Can you work these out from the model? Positions are in its coordinate system, mm. A direction names the side the tool comes from. Give positions to 0.01 mm unless a question says otherwise; leave off trailing zeros. Loops run counter-clockwise (first coordinate to the right, second up) from the corner with the lowest first, then second, coordinate; pieces in that order, holes last. Notation, with made-up numbers: (62, 7.25) -> (91, 7.25) arc R17 ccw to (91, 16.25) -> close; hole circle Ø9 at (71.25, 30). An arc over 180 degrees is marked (long way). Return JSON: item names as keys, results as strings. Group by question number.
Q1. Which directions (+Z, -Z, +X, -X, +Y, -Y) give clear straight access to the entire face, cutting with the end or side of a thin tool? Please do faces 5 (the cylindrical face through (-36.495, 3.486, -27.382)), 6 (the flat face through (0, 3, 36.5)), 7 (the flat face through (-18.958, 2.282, 1.44)), 8 (the cylindrical face through (17.29, 3.49, 33.04)).
Q2. I need wall thicknesses on line 1 along Z through (x, y) = (6, 4.3); line 2 along Z through (x, y) = (-15.5, 2.25); line 3 along Y through (x, z) = (-44, -10.5). Which ranges of each line are inside material? Lowest first, please. Write a range as [from, to].
Q3. Thinking about a two-plate mould opening in X: for faces 1 (the flat face through (0, 3, -36.5)), 2 (the cylindrical face through (33.535, 2.218, -19.087)), 3 (the cylindrical face through (18.945, 2.218, 19.066)), 4 (the flat face through (40.18, 0.74, -0.58)), which applies, pulls with the +X half, pulls with the -X half, needs draft (parallel to the pull), parting line crosses it, or undercut?
Q4. Suppose I cut it at C-C, the plane z = -17.5. Please give me the cut outline in (x, y), and give its area (3 significant figures).
Q5. Suppose I cut it at B-B, the plane y = 3.8. Please give me the cut outline in (x, z).
Q6. Suppose I cut it at A-A, the plane x = 4.5. Please give me the cut outline in (y, z), and give its area (3 significant figures).
Q7. Suppose I cut it at D-D, the plane z = 6.5. Please give me the cut outline in (x, y), and give its area (3 significant figures).
Q8. Will these pins go through, and if not, where does the flat tip stop? pin 1 (1 mm diameter, centred on x = 29.5, y = 4, fed in from +Z); pin 2 (2.5 mm diameter, centred on x = -6, y = 3, fed in from -Z); pin 3 (2 mm diameter, centred on y = 3, z = 3, fed in from -X).
Autodesk Inventor part; units mm, degrees
ref_plane "YZ Plane" through (0, 0, 0) normal (1, 0, 0) x (0, 1, 0)
ref_plane "XZ Plane" through (0, 0, 0) normal (0, 1, 0) x (-1, 0, 0)
ref_plane "XY Plane" through (0, 0, 0) normal (0, 0, 1) x (1, 0, 0)
sketch "Skizze1" plane through (0, 0, 0) normal (0, 1, 0) x (-1, 0, 0)
  line L0 (-22.75, 41.5) -> (22.75, 41.5)
  line L1 (22.75, 41.5) -> (57.1297, -41.5)
  line L2 (57.1297, -41.5) -> (-57.1297, -41.5)
  line L3 (-57.1297, -41.5) -> (-22.75, 41.5)
  line L4 (79.9816, 0) -> (-79.9816, 0) construction
  line L5 (0, -58.1) -> (0, 58.1) construction
  point P0 (0, 0)
  dimension "d0" = 83
  dimension "d1" = 112.5
  dimension "d2" = 45.5
extrude "Extrusion1" add sketch "Skizze1" along normal blind 6
sketch "Skizze2" plane through (0, 6, 0) normal (0, 1, 0) x (1, 0, 0)
  line L0 (-22.75, -41.5) -> (22.75, -41.5)
  line L1 (22.75, -41.5) -> (57.1297, 41.5)
  line L2 (57.1297, 41.5) -> (-57.1297, 41.5)
  line L3 (-57.1297, 41.5) -> (-22.75, -41.5)
  line L4 (-49.6467, 36.5) -> (49.6467, 36.5)
  line L5 (49.6467, 36.5) -> (19.4091, -36.5)
  line L6 (19.4091, -36.5) -> (-19.4091, -36.5)
  line L7 (-19.4091, -36.5) -> (-49.6467, 36.5)
  point P0 (0, 0)
  dimension "d5" = 5
extrude "Extrusion2" cut sketch "Skizze2" against normal blind 3.5
sketch "Skizze4" plane through (0, 6, 0) normal (0, 1, 0) x (1, 0, 0)
  line L0 (58.5766, 41.5) -> (-55.8797, 41.5) construction
  line L1 (-55.8797, 41.5) -> (-21.5, -41.5) construction
  line L2 (-21.5, -41.5) -> (24.1969, -41.5) construction
  line L3 (57.1297, 41.5) -> (22.75, -41.5) construction
  line L4 (22.4292, -40.7678) -> (56.8089, 42.2322) construction
  line L5 (-29.4207, 23.8207) -> (30.0466, 23.8207)
  line L6 (30.0466, 23.8207) -> (10.313, -23.8207)
  line L7 (10.313, -23.8207) -> (-9.687, -23.8207)
  line L8 (-9.687, -23.8207) -> (-29.4207, 23.8207)
  point P0 (0, 0)
  dimension "d15" = 20
extrude "Extrusion3" cut sketch "Skizze4" against normal through all
fillet "Rundung1" radius 3 4 edges at (30.0466, 3, -23.8207) (10.313, 3, 23.8207) (-9.687, 3, 23.8207) (-29.4207, 3, -23.8207)
sketch "Skizze5" plane through (0, 6, 0) normal (0, 1, 0) x (1, 0, 0)
  line L0 (-10.4541, -21.9687) -> (-27.7025, 19.6726)
  arc A0 (-24.9309, 23.8207) -> (-27.7025, 19.6726) centre (-24.9309, 20.8207) ccw
  line L1 (-24.9309, 23.8207) -> (25.5568, 23.8207)
  arc A1 (28.3284, 19.6726) -> (25.5568, 23.8207) centre (25.5568, 20.8207) ccw
  line L2 (28.3284, 19.6726) -> (11.0801, -21.9687)
  arc A2 (8.3084, -23.8207) -> (11.0801, -21.9687) centre (8.3084, -20.8207) ccw
  line L3 (8.3084, -23.8207) -> (-7.6825, -23.8207)
  arc A3 (-10.4541, -21.9687) -> (-7.6825, -23.8207) centre (-7.6825, -20.8207) ccw
  line L4 (-49.6467, 36.5) -> (-19.4091, -36.5)
  line L5 (-19.4091, -36.5) -> (19.4091, -36.5)
  line L6 (19.4091, -36.5) -> (49.6467, 36.5)
  line L7 (49.6467, 36.5) -> (-49.6467, 36.5)
  point P0 (0, 0)
extrude "Extrusion4" cut sketch "Skizze5" against normal blind 0.5
sketch "Skizze6" plane through (0, 5.5, 0) normal (0, 1, 0) x (1, 0, 0)
  circle A0 centre (-32.1216, 17.5) radius 4.7 construction
  circle A1 centre (-16.7957, -19.5) radius 4.7 construction
  circle A2 centre (16.9926, -19.5) radius 4.7 construction
  circle A3 centre (32.3185, 17.5) radius 4.7 construction
  line L0 (-24.9683, -43.2) -> (25.1652, -43.2) construction
  line L1 (25.1652, -43.2) -> (61.3675, 44.2) construction
  line L2 (61.3675, 44.2) -> (11.1438, 44.2) construction
  arc A4 (11.1438, 44.2) -> (-10.9469, 44.2) centre (0.0985, 34.5) ccw construction
  line L3 (-10.9469, 44.2) -> (-61.1705, 44.2) construction
  line L4 (-61.1705, 44.2) -> (-24.9683, -43.2) construction
  point P0 (0, 0)
  point P1 (-32.1216, 17.5)
  point P2 (-16.7957, -19.5)
  point P3 (16.9926, -19.5)
  point P4 (32.3185, 17.5)
hole "Bohrung2" at (-32.1216, 5.5, -17.5) at (-16.7957, 5.5, 19.5) at (16.9926, 5.5, 19.5) at (32.3185, 5.5, -17.5) direction (0, -1, 0) diameter 4 depth 8 tip angle 118
sketch "Skizze7" plane through (0, 5.5, 0) normal (0, 1, 0) x (1, 0, 0)
  circle A0 centre (16.9926, -19.5) radius 2
  circle A1 centre (-32.1216, 17.5) radius 2
  circle A2 centre (-16.7957, -19.5) radius 2
  circle A3 centre (32.3185, 17.5) radius 2
  arc A4 (-10.4541, -21.9687) -> (-7.6825, -23.8207) centre (-7.6825, -20.8207) ccw
  line L0 (-27.7025, 19.6726) -> (-10.4541, -21.9687)
  arc A5 (-24.9309, 23.8207) -> (-27.7025, 19.6726) centre (-24.9309, 20.8207) ccw
  line L1 (25.5568, 23.8207) -> (-24.9309, 23.8207)
  arc A6 (28.3284, 19.6726) -> (25.5568, 23.8207) centre (25.5568, 20.8207) ccw
  line L2 (11.0801, -21.9687) -> (28.3284, 19.6726)
  arc A7 (8.3084, -23.8207) -> (11.0801, -21.9687) centre (8.3084, -20.8207) ccw
  line L3 (-7.6825, -23.8207) -> (8.3084, -23.8207)
  line L4 (-19.4091, -36.5) -> (-49.6467, 36.5)
  line L5 (19.4091, -36.5) -> (-19.4091, -36.5)
  line L6 (49.6467, 36.5) -> (19.4091, -36.5)
  line L7 (-49.6467, 36.5) -> (49.6467, 36.5)
  point P0 (0, 0)
extrude "Extrusion5" cut sketch "Skizze7" against normal blind 1
fillet "Rundung2" radius 20 4 edges at (-19.4091, 3.5, 36.5) (19.4091, 3.5, 36.5) (49.6467, 3.5, -36.5) (-49.6467, 3.5, -36.5)
sketch "Skizze8" plane through (0, 2.5, 0) normal (0, 1, 0) x (1, 0, 0)
  line L0 (19.7146, 36.5) -> (-19.7146, 36.5)
  arc A0 (38.1922, 8.8463) -> (19.7146, 36.5) centre (19.7146, 16.5) ccw
  line L1 (24.5231, -24.1537) -> (38.1922, 8.8463)
  arc A1 (6.0455, -36.5) -> (24.5231, -24.1537) centre (6.0455, -16.5) ccw
  line L2 (-6.0455, -36.5) -> (6.0455, -36.5)
  arc A2 (-24.5231, -24.1537) -> (-6.0455, -36.5) centre (-6.0455, -16.5) ccw
  line L3 (-38.1922, 8.8463) -> (-24.5231, -24.1537)
  arc A3 (-19.7146, 36.5) -> (-38.1922, 8.8463) centre (-19.7146, 16.5) ccw
  line L4 (22.75, -41.5) -> (-22.75, -41.5)
  line L5 (57.1297, 41.5) -> (22.75, -41.5)
  line L6 (-57.1297, 41.5) -> (57.1297, 41.5)
  line L7 (-22.75, -41.5) -> (-57.1297, 41.5)
  point P0 (0, 0)
extrude "Extrusion6" cut sketch "Skizze8" against normal blind 1
properties part number "Stage2" material "ABS-Kunststoff"
Ans:
{
 "1": {"face 5": "-X, +Y", "face 6": "+Z, +X, -X, +Y", "face 7": "+Y, -Y", "face 8": "+Z, +X, +Y"},
 "2": {"line 1": "z = [-36.5, -23.82], [23.82, 36.5]", "line 2": "z = [-36.5, -23.82], [9.79, 17.98], [21.02, 34.12]", "line 3": "y = [0, 1.5]"},
 "3": {"face 1": "needs draft", "face 2": "undercut", "face 3": "undercut", "face 4": "pulls with the +X half"},
 "4": {"outline": "(-47.19, 0) -> (-34.12, 0) -> (-34.12, 4.5) -> (-39.69, 4.5) -> (-39.69, 1.5) -> (-47.19, 1.5) -> close; (-30.12, 0) -> (-26.8, 0) -> (-26.8, 4.5) -> (-30.12, 4.5) -> close; (27.43, 0) -> (30.32, 0) -> (30.32, 4.5) -> (27.43, 4.5) -> close; (34.32, 0) -> (47.19, 0) -> (47.19, 1.5) -> (39.69, 1.5) -> (39.69, 4.5) -> (34.32, 4.5) -> close", "area": "99.7 mm^2"},
 "5": {"outline": "(-38.19, -8.85) arc R20 ccw to (-19.71, -36.5) -> (19.71, -36.5) arc R20 ccw to (38.19, -8.85) -> (24.52, 24.15) arc R20 ccw to (6.05, 36.5) -> (-6.05, 36.5) arc R20 ccw to (-24.52, 24.15) -> close; hole circle Ø4 at (-32.12, -17.5); hole (-27.7, -19.67) arc R3 ccw to (-24.93, -23.82) -> (25.56, -23.82) arc R3 ccw to (28.33, -19.67) -> (11.08, 21.97) arc R3 ccw to (8.31, 23.82) -> (-7.68, 23.82) arc R3 ccw to (-10.45, 21.97) -> close; hole circle Ø4 at (-16.8, 19.5); hole circle Ø4 at (16.99, 19.5); hole circle Ø4 at (32.32, -17.5)"},
 "6": {"outline": "(0, -41.5) -> (1.5, -41.5) -> (1.5, -36.5) -> (4.5, -36.5) -> (4.5, -23.82) -> (0, -23.82) -> close; (0, 23.82) -> (4.5, 23.82) -> (4.5, 36.5) -> (1.5, 36.5) -> (1.5, 41.5) -> (0, 41.5) -> close", "area": "129 mm^2"},
 "7": {"outline": "(-37.25, 0) -> (-16.86, 0) -> (-16.86, 4.5) -> (-31.84, 4.5) -> (-31.84, 1.5) -> (-37.25, 1.5) -> close; (17.49, 0) -> (37.25, 0) -> (37.25, 1.5) -> (31.84, 1.5) -> (31.84, 4.5) -> (17.49, 4.5) -> close", "area": "148 mm^2"},
 "8": {"pin 1": "stops at z = 13.35", "pin 2": "stops at z = -36.5", "pin 3": "stops at x = -33.7"}
}
